Check sheet for the modelled part. Datum: model origin and axes. Units: mm. Coordinates: 2 decimals unless noted, no trailing zeros. Loops run counter-clockwise (first coordinate to the right, second up) from the corner with the lowest first, then second, coordinate; pieces in that order, holes last. Notation, with made-up numbers: (50, 73) - (56, 73) arc R25 ccw to (56, 96) - close; hole circle Ø3 at (-19, -20). An arc over 180 degrees is marked (long way). Use a Markdown table: item, result. Add a question column.
1) Go/stop test with a flat-tipped pin: P1, Ø13.5, axis at x = 30, z = -40, coming from the -Y side. Record where the tip stops, or that it passes through.
2) Sectioned sample at B-B, the plane z = -55. State how many separate pieces and enclosed holes the cut face has, then the cut area to 3 significant figures.
3) Thickness scan on line 1 (Z direction, x = 30, y = 1.15); line 2 (Z direction, x = 120.5, y = 2.6). Record the ranges inside material, lowest first.
4) Sectioned sample at A-A, the plane x = 10. Enter the section's corners in (y, z).
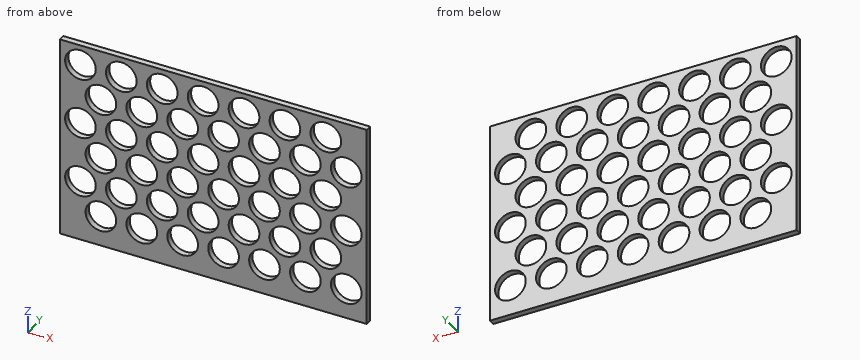
from build123d import *

# Parameters (mm, degrees)
SKETCH_1_W          = 150
SKETCH_1_H          = 100
EXTRUDE_1_DEPTH     = 3
SKETCH_2_R          = 7.5
CUT_EXTRUDE_1_DEPTH = 4


with BuildPart() as part:
    # Эскиз1 → Бобышка-Вытянуть1 (new body)
    with BuildSketch(Plane(origin=(0, 0, 0), x_dir=(1, 0, 0), z_dir=(0, 1, 0))):
        with Locations((75, 50)):
            Rectangle(SKETCH_1_W, SKETCH_1_H)
    extrude(amount=EXTRUDE_1_DEPTH)

    # Эскиз2 → Вырез-Вытянуть1 (cut, through all)
    with BuildSketch(Plane(origin=(0, 3, 0), x_dir=(1, 0, 0), z_dir=(0, 1, 0))):
        with Locations((10, 10)):
            Circle(SKETCH_2_R)
        with Locations((20, 25)):
            Circle(SKETCH_2_R)
        with Locations((30, 10)):
            Circle(SKETCH_2_R)
        with Locations((40, 25)):
            Circle(SKETCH_2_R)
        with Locations((50, 10)):
            Circle(SKETCH_2_R)
        with Locations((60, 25)):
            Circle(SKETCH_2_R)
        with Locations((70, 10)):
            Circle(SKETCH_2_R)
        with Locations((80, 25)):
            Circle(SKETCH_2_R)
        with Locations((90, 10)):
            Circle(SKETCH_2_R)
        with Locations((100, 25)):
            Circle(SKETCH_2_R)
        with Locations((110, 10)):
            Circle(SKETCH_2_R)
        with Locations((120, 25)):
            Circle(SKETCH_2_R)
        with Locations((130, 10)):
            Circle(SKETCH_2_R)
        with Locations((140, 25)):
            Circle(SKETCH_2_R)
        with Locations((30, 40)):
            Circle(SKETCH_2_R)
        with Locations((40, 55)):
            Circle(SKETCH_2_R)
        with Locations((50, 40)):
            Circle(SKETCH_2_R)
        with Locations((60, 55)):
            Circle(SKETCH_2_R)
        with Locations((70, 40)):
            Circle(SKETCH_2_R)
        with Locations((80, 55)):
            Circle(SKETCH_2_R)
        with Locations((90, 40)):
            Circle(SKETCH_2_R)
        with Locations((100, 55)):
            Circle(SKETCH_2_R)
        with Locations((110, 40)):
            Circle(SKETCH_2_R)
        with Locations((120, 55)):
            Circle(SKETCH_2_R)
        with Locations((130, 40)):
            Circle(SKETCH_2_R)
        with Locations((140, 55)):
            Circle(SKETCH_2_R)
        with Locations((30, 70)):
            Circle(SKETCH_2_R)
        with Locations((40, 85)):
            Circle(SKETCH_2_R)
        with Locations((50, 70)):
            Circle(SKETCH_2_R)
        with Locations((60, 85)):
            Circle(SKETCH_2_R)
        with Locations((70, 70)):
            Circle(SKETCH_2_R)
        with Locations((80, 85)):
            Circle(SKETCH_2_R)
        with Locations((90, 70)):
            Circle(SKETCH_2_R)
        with Locations((100, 85)):
            Circle(SKETCH_2_R)
        with Locations((110, 70)):
            Circle(SKETCH_2_R)
        with Locations((120, 85)):
            Circle(SKETCH_2_R)
        with Locations((130, 70)):
            Circle(SKETCH_2_R)
        with Locations((140, 85)):
            Circle(SKETCH_2_R)
        with Locations((10, 40)):
            Circle(SKETCH_2_R)
        with Locations((20, 55)):
            Circle(SKETCH_2_R)
        with Locations((10, 70)):
            Circle(SKETCH_2_R)
        with Locations((20, 85)):
            Circle(SKETCH_2_R)
    extrude(amount=-CUT_EXTRUDE_1_DEPTH, mode=Mode.SUBTRACT)


solid = part.part
Solved:
| question | item | result |
|---|---|---|
| 1 | P1 | passes through |
| 2 | separate pieces | 8 |
| 2 | enclosed holes | 0 |
| 2 | area | 135 mm2 |
| 3 | line 1 | z = -100 to -77.5, -62.5 to -47.5, -32.5 to -17.5, -2.5 to 0 |
| 3 | line 2 | z = -100 to -92.48, -77.52 to -62.48, -47.52 to -32.48, -17.52 to 0 |
| 4 | outline | (0, -100) - (3, -100) - (3, -77.5) - (0, -77.5) - close; (0, -62.5) - (3, -62.5) - (3, -47.5) - (0, -47.5) - close; (0, -32.5) - (3, -32.5) - (3, -17.5) - (0, -17.5) - close; (0, -2.5) - (3, -2.5) - (3, 0) - (0, 0) - close |
